Read the model definition and answer for the solid it produces. Units are mm, in the model's axes. A direction names the side the tool comes from. Round coordinates to 2 decimals unless told otherwise and drop trailing zeros. Order: outer loops, then holes, each group sorted by start corner. A loop starts at its lowest first (then second) coordinate and runs counter-clockwise, first axis right, second up. Notation, with made-up numbers: (-8, 67.25) -> (2, 67.25) arc R9 ccw to (2, 71.25) -> close; hole circle Ø7 at (69, -35.5). An arc over 180 degrees is marked (long way). Use a Markdown table: item, result. Add a question column.
1. Section D-D, the plane z = 1.25 is taken. Give the vertices of the cut face in (x, y).
2. Section B-B, the plane z = 14 is taken. Give the vertices of the cut face in (x, y) (3 decimals), then the cut area to 3 significant figures.
3. For faces 4 (the face through (0, -18, 0)), 5 (the face through (13.887, -10.648, 1.479)), 6 (the face through (-12.358, -9.024, 11.5)), determine the directions among +Z, -Z, +X, -X, +Y, -Y from which every point of the face is accessible in a straight line to the end or side of a thin tool.
4. Section C-C, the plane x = 10.5 is taken. Give the vertices of the cut face in (y, z).
5. Section A-A, the plane y = 0 is taken. Give the vertices of the cut face in (x, z), then the cut area to 3 significant figures.
6. The mould has two halves that part along X. Classify faces 1 (the face through (-12.92, 5.85, 11.5)), 2 (the face through (-5, 9, 15)), 3 (the face through (-4.336, -19.524, 7.395)): +X half, -X half, draft (parallel to the pull), parting line (faces both ways), or undercut.
7. Given pin 1 (2 mm diameter, centred on x = 0, y = -15, fed in from -Z); pin 2 (2 mm diameter, centred on x = -3, z = 5, fed in from +Y); pin 3 (3 mm diameter, centred on x = 10, z = 8, fed in from -Y), each flat-ended and moving along its own axis, determine where each tip first touches the part or whether it passes through.
8. Consider L1, parallel to Y at x = 13, z = 9.75; L2, parallel to Y at x = -0.5, z = 13.75; L3, parallel to Z at x = -4, y = 13. Determine where each line is inside the solid, lowest interval first. Write a range as [from, to].
```python
from build123d import *

# Parameters (mm, degrees)
SKETCH1_R           = 20
BOSS_EXTRUDE1_DEPTH = 15
SKETCH2_R           = 10
CUT_EXTRUDE1_DEPTH  = 5
CIRPATTERN2_COUNT   = 6
SKETCH5_R           = 17.5
CUT_EXTRUDE2_DEPTH  = 3


with BuildPart() as part:
    # Sketch1 → Boss-Extrude1 (new body)
    with BuildSketch(Plane.XY):
        Circle(SKETCH1_R)
    extrude(amount=BOSS_EXTRUDE1_DEPTH)

    # Sketch2 → Cut-Extrude1 (cut)
    with BuildSketch(Plane.XY.offset(15)):
        Circle(SKETCH2_R)
    extrude(amount=-CUT_EXTRUDE1_DEPTH, mode=Mode.SUBTRACT)

    # Sketch4 → M4x0.7 Tapped Hole1 (revolve, cut)
    with BuildSketch(Plane(origin=(0, 15, 15), x_dir=(0, -1, 0), z_dir=(1, 0, 0))):
        Polygon((0, 0), (0, 8.091420021), (1.65, 7.1), (1.65, 0), align=None)
    m4x0_7_tapped_hole1 = revolve(axis=Axis((0, 15, 21.35), (0, 0, -1)), mode=Mode.SUBTRACT)

    # CirPattern2: M4x0.7 Tapped Hole1 ×6 about axis
    cirpattern2_axis = Axis((0, 0, 0), (0, 0, 1))
    for i in range(1, CIRPATTERN2_COUNT):
        add(m4x0_7_tapped_hole1.rotate(cirpattern2_axis, i * 360 / CIRPATTERN2_COUNT), mode=Mode.SUBTRACT)

    # Sketch5 → Cut-Extrude2 (cut)
    with BuildSketch(Plane(origin=(0, 0, 0), x_dir=(-1, 0, 0), z_dir=(0, 0, -1))):
        Circle(SKETCH5_R)
    extrude(amount=-CUT_EXTRUDE2_DEPTH, mode=Mode.SUBTRACT)


solid = part.part
```
Verdict:
| question | item | result |
|---|---|---|
| 1 | outline | circle Ø40 at (0, 0); hole circle Ø35 at (0, 0) |
| 2 | outline | circle Ø40 at (0, 0); hole circle Ø3.3 at (-12.99, -7.5); hole circle Ø3.3 at (-12.99, 7.5); hole circle Ø20 at (0, 0); hole circle Ø3.3 at (0, -15); hole circle Ø3.3 at (0, 15); hole circle Ø3.3 at (12.99, -7.5); hole circle Ø3.3 at (12.99, 7.5) |
| 2 | area | 891 mm2 |
| 3 | face 4 | -Z, +X, -X, +Y, -Y |
| 3 | face 5 | -Z |
| 3 | face 6 | +Z |
| 4 | outline | (-17.02, 0) -> (-14, 0) -> (-14, 3) -> (14, 3) -> (14, 0) -> (17.02, 0) -> (17.02, 15) -> (-17.02, 15) -> close |
| 5 | outline | (-20, 0) -> (-17.5, 0) -> (-17.5, 3) -> (17.5, 3) -> (17.5, 0) -> (20, 0) -> (20, 15) -> (10, 15) -> (10, 10) -> (-10, 10) -> (-10, 15) -> (-20, 15) -> close |
| 5 | area | 395 mm2 |
| 6 | face 1 | undercut |
| 6 | face 2 | draft |
| 6 | face 3 | parting line |
| 7 | pin 1 | stops at z = 3 |
| 7 | pin 2 | stops at y = 19.9 |
| 7 | pin 3 | stops at y = -18.1 |
| 8 | L1 | y = [-15.2, -9.15], [-5.85, 5.85], [9.15, 15.2] |
| 8 | L2 | y = [-19.99, -16.57], [-13.43, -9.99], [9.99, 13.43], [16.57, 19.99] |
| 8 | L3 | z = [3, 15] |
